The listing builds one solid part. Answer for the finished solid, in the listing's coordinates (mm). A direction names the side the tool comes from. Coordinates: 2 decimals unless noted, no trailing zeros. Order: outer loops, then holes, each group sorted by start corner. A loop starts at its lowest first (then second) coordinate and runs counter-clockwise, first axis right, second up. Notation, with made-up numbers: (2, 14) - (51, 14) arc R28 cw to (51, 43) - close; hole circle Ø6 at (-4.5, 54). An arc over 180 degrees is marked (long way). Use one line per item in the form item = value. Start each with the question number.
Item 1: Section A-A, the plane y = -27 is taken. Write down the section's boundary in (x, z) (3 decimals), and give its area (3 significant figures).
Item 2: Section C-C, the plane z = -4.5 is taken. Write down the section's boundary in (x, y) (3 decimals).
Item 3: Section B-B, the plane x = -2 is taken. Write down the section's boundary in (y, z) (3 decimals), and give its area (3 significant figures).
Item 4: Consider line 1 along Z through (x, y) = (-4, -27) (3 decimals); line 2 along Y through (x, z) = (-10.75, 10.5) (3 decimals); line 3 along X through (y, z) = (-18.5, 0.5). Determine where each line is inside the solid, lowest interval first. Write a range as [from, to].
Item 5: The mould has two halves that part along Z. Classify faces 4 (the flat face through (-12, 6, 0)), 5 (the cylindrical face through (-6.67, -40.27, 20.45)), 6 (the flat face through (-6, -16, 17.875)): released by +Z, released by -Z, zero draft, split by the parting line, or undercut.
Item 6: Each of these flat-tipped pins is pushed along its axis until it touches: pin 1 Ø6 at (x, z) = (-8, -10.5) entering from +Y; pin 2 Ø18 at (y, z) = (-27, 0.5) entering from +X; pin 3 Ø2 at (x, y) = (-7.5, -37) entering from -Z. Where does it stop, or does it pass through?
Item 7: A tool of negligible diameter and unlimited length cuts with its end or side. For faces 1 (the cylindrical face through (-5.65, 3.59, 17.09)), 2 (the flat face through (-6, -37.875, 0)), 3 (the flat face through (-13.15, -19, 0)), from which of +Z, -Z, +X, -X, +Y, -Y can it reach the whole face along a straight path? Write none if from no direction.
Item 8: Section D-D, the plane y = 2 is taken. Write down the section's boundary in (x, z).
from build123d import *

# Parameters (mm, degrees)
BOSS_EXTRUDE1_START = -13.15
BOSS_EXTRUDE1_DEPTH = 2
BOSS_EXTRUDE2_START = -11.15
BOSS_EXTRUDE2_DEPTH = 11.15


with BuildPart() as part:
    # Sketch2 → Boss-Extrude1 (new body)
    with BuildSketch(Plane(origin=(0, 0, 0), x_dir=(0, 0, -1), z_dir=(1, 0, 0)).offset(BOSS_EXTRUDE1_START)):
        with BuildLine():
            Line((14.561593319, 6), (-14.561593319, 6))
            ThreePointArc((-14.561593319, 6), (-19.647313485, 2.405871392), (-23.875, -2.166762072))
            Line((-23.875, -2.166762072), (-23.875, -31.875))
            ThreePointArc((-23.875, -31.875), (-20.360281374, -40.360281374), (-11.875, -43.875))
            Line((-11.875, -43.875), (11.875, -43.875))
            ThreePointArc((11.875, -43.875), (20.360281374, -40.360281374), (23.875, -31.875))
            Line((23.875, -31.875), (23.875, -2.166762072))
            ThreePointArc((23.875, -2.166762072), (19.647313485, 2.405871392), (14.561593319, 6))
        make_face()
    extrude(amount=BOSS_EXTRUDE1_DEPTH)

    # Sketch2<3> → Boss-Extrude2 (add)
    with BuildSketch(Plane(origin=(0, 0, 0), x_dir=(0, 0, -1), z_dir=(1, 0, 0)).offset(BOSS_EXTRUDE2_START)):
        with BuildLine():
            ThreePointArc((17, 4.475293665), (15.948645849, 5.173015226), (14.868697479, 5.825604258))
            ThreePointArc((14.868697479, 5.825604258), (17.069332723, 3.628967773), (17.875, 0.625818166))
            Line((17.875, 0.625818166), (17.875, -31.875))
            ThreePointArc((17.875, -31.875), (16.117640687, -36.117640687), (11.875, -37.875))
            Line((11.875, -37.875), (-11.875, -37.875))
            ThreePointArc((-11.875, -37.875), (-16.117640687, -36.117640687), (-17.875, -31.875))
            Line((-17.875, -31.875), (-17.875, 0.625818166))
            ThreePointArc((-17.875, 0.625818166), (-17.069332723, 3.628967773), (-14.868697479, 5.825604258))
            ThreePointArc((-14.868697479, 5.825604258), (-15.948645849, 5.173015226), (-17, 4.475293665))
            ThreePointArc((-17, 4.475293665), (-20.70557008, 1.431737392), (-23.875, -2.166762072))
            Line((-23.875, -2.166762072), (-23.875, -31.875))
            ThreePointArc((-23.875, -31.875), (-20.360281374, -40.360281374), (-11.875, -43.875))
            Line((-11.875, -43.875), (11.875, -43.875))
            ThreePointArc((11.875, -43.875), (20.360281374, -40.360281374), (23.875, -31.875))
            Line((23.875, -31.875), (23.875, -2.166762072))
            ThreePointArc((23.875, -2.166762072), (20.70557008, 1.431737392), (17, 4.475293665))
        make_face()
    extrude(amount=BOSS_EXTRUDE2_DEPTH)


solid = part.part
Response:
q1.outline = (-13.15, -23.875) - (0, -23.875) - (0, -17.875) - (-11.15, -17.875) - (-11.15, 17.875) - (0, 17.875) - (0, 23.875) - (-13.15, 23.875) - close
q1.area = 229 mm2
q2.outline = (-13.15, -43.875) - (0, -43.875) - (0, -37.875) - (-11.15, -37.875) - (-11.15, 6) - (-13.15, 6) - close
q3.outline = (-43.875, -11.875) arc R12 ccw to (-31.875, -23.875) - (-2.167, -23.875) arc R29.8 ccw to (5.826, -14.869) arc R6 cw to (0.626, -17.875) - (-31.875, -17.875) arc R6 cw to (-37.875, -11.875) - (-37.875, 11.875) arc R6 cw to (-31.875, 17.875) - (0.626, 17.875) arc R6 cw to (5.826, 14.869) arc R29.8 ccw to (-2.167, 23.875) - (-31.875, 23.875) arc R12 ccw to (-43.875, 11.875) - close
q3.area = 712 mm2
q4.line_1 = [-23.875, -17.875], [17.875, 23.875]
q4.line_2 = [-43.875, -37.875]
q4.line_3 = [-13.15, -11.15]
q5.face_4 = zero draft
q5.face_5 = released by +Z
q5.face_6 = undercut
q6.pin_1 = -37.65
q6.pin_2 = -11.15
q6.pin_3 = -23.14
q7.face_1 = +X
q7.face_2 = +X, +Y
q7.face_3 = +Z, -Z, -X, +Y, -Y
q8.outline = (-13.15, -20.1) - (0, -20.1) - (0, -17.72) - (-11.15, -17.72) - (-11.15, 17.72) - (0, 17.72) - (0, 20.1) - (-13.15, 20.1) - close
